from build123d import *

# Parameters (mm, degrees)
SKETCH_1_R      = 20
EXTRUDE_1_DEPTH = 150
SKETCH_3_R      = 10
EXTRUDE_2_DEPTH = 40


with BuildPart() as part:
    # 草图1 → 凸台-拉伸1 (new, symmetric)
    with BuildSketch(Plane.XY):
        Circle(SKETCH_1_R)
    extrude(amount=EXTRUDE_1_DEPTH, both=True)

    # 草图3 → 凸台-拉伸2 (add)
    with BuildSketch(Plane(origin=(0, 0, 0), x_dir=(1, 0, 0), z_dir=(0, 1, 0))):
        with Locations(Location((0, 126.551526586, 0), (0, 0, 90))):
            Circle(SKETCH_3_R)
        with Locations(Location((0, -126.551526586, 0), (0, 0, 90))):
            Circle(SKETCH_3_R)
    extrude(amount=EXTRUDE_2_DEPTH)


solid = part.part
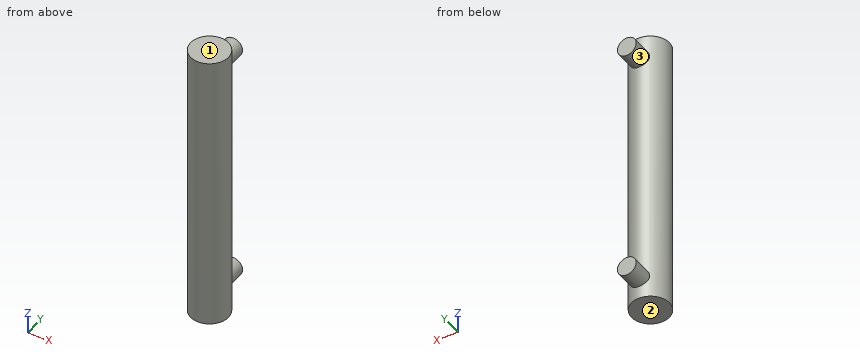
Build history of the part. All positions in model axes, mm. Face numbers are marked on the shaded views. Round coordinates to 2 decimals unless told otherwise and drop trailing zeros. Write each loop counter-clockwise with the first axis right and the second up, starting at its lowest first coordinate (ties: lowest second). Pieces come first, ordered by that corner, then holes. Notation, with made-up numbers: M 35,32.5 L 44,32.5 A16 ccw 44,62.5 Z; hole C 11.25,-39.75 d8. An arc over 180 degrees is marked long. Use CSV: the item, a comma, the result in double quotes.
1. Wall check: probe 1 along Z at (x, y) = (5, 26.5); probe 2 along Z at (x, y) = (8, 24); probe 3 along Y at (x, z) = (-17, -8). Give the ranges that are in metal, low to high. Write a range as from..to.
Reply:
probe 1,"z = -135.21..-117.89, 117.89..135.21"
probe 2,"z = -132.55..-120.55, 120.55..132.55"
probe 3,"y = -10.54..10.54"
2. Saw through at B-B (x = 0). Give the cut face in (y, z), plus the area to 3 significant figures.
Reply:
outline,"M -20,-150 L 20,-150 L 20,-136.55 L 40,-136.55 L 40,-116.55 L 20,-116.55 L 20,116.55 L 40,116.55 L 40,136.55 L 20,136.55 L 20,150 L -20,150 Z"
area,"12,800 mm²"
3. Saw through at D-D (y = 11.5). Give the cut face in (x, z).
Reply:
outline,"M -16.36,-150 L 16.36,-150 L 16.36,150 L -16.36,150 Z"
4. Saw through at A-A (y = 27.5). Give the cut face in (x, z), plus the area to 3 significant figures.
Reply:
outline,"C 0,-126.55 d20; C 0,126.55 d20"
area,"628 mm²"
5. Two-plate mould, pull along Z, no slides. Class the marked faces 1, 2 and 3: +Z half, -Z half, draft (parallel to the pull), parting line (faces both ways), or undercut.
Reply:
face 1,"+Z half"
face 2,"-Z half"
face 3,"undercut"
6. Flat gauge pins, fed straight in: pin 1 (1.5 mm diameter, centred on x = -7.5, z = -80.5, fed in from +Y); pin 2 (12 mm diameter, centred on y = -7, z = -37.5, fed in from +X) (3 decimals); pin 3 (10 mm diameter, centred on y = -14, z = 89, fed in from -X). Where does each tip first touch, or does it go through?
Reply:
pin 1,"stops at y = 18.83"
pin 2,"stops at x = 19.975"
pin 3,"stops at x = -17.86"
7. Saw through at C-C (z = 26.5). Give the cut face in (x, y), plus the area to 3 significant figures.
Reply:
outline,"C 0,0 d40"
area,"1,260 mm²"
